Geometry check sheet. Reference: the model listing, model coordinates, mm. Give positions to 0.01 mm unless a question says otherwise; leave off trailing zeros. Loops run counter-clockwise (first coordinate to the right, second up) from the corner with the lowest first, then second, coordinate; pieces in that order, holes last. Notation, with made-up numbers: (86, 57) -> (136, 57) arc R31 ccw to (136, 89) -> close; hole circle Ø1 at (14, 29.5). An arc over 180 degrees is marked (long way). One line per question, with ' | ' between items.
from build123d import *

# Parameters (mm, degrees)
ESBO_O1_W                = 150
ESBO_O1_H                = 40
ESBO_O1_R                = 2.5
ESBO_O1_R_2              = 6
RESSALTO_EXTRUS_O1_DEPTH = 12.7
ESBO_O4_R                = 5.5
CORTE_EXTRUS_O1_DEPTH    = 8
ESBO_O7_W                = 150
ESBO_O7_H                = 10
RESSALTO_EXTRUS_O4_DEPTH = 12.7
ESBO_O8_W                = 10
ESBO_O8_H                = 50
RESSALTO_EXTRUS_O5_DEPTH = 12.7
ESBO_O9_R                = 2
CORTE_EXTRUS_O2_DEPTH    = 10


with BuildPart() as part:
    # Esboço1 → Ressalto-extrusão1 (new body)
    with BuildSketch(Plane(origin=(0, 0, 0), x_dir=(1, 0, 0), z_dir=(0, 1, 0))):
        Rectangle(ESBO_O1_W, ESBO_O1_H)
        with Locations(Location((0, 0, 0), (0, 0, 270))):
            Circle(ESBO_O1_R, mode=Mode.SUBTRACT)
        with Locations(Location((-57.5, 0, 0), (0, 0, 270))):
            Circle(ESBO_O1_R_2, mode=Mode.SUBTRACT)
        with Locations(Location((57.5, 0, 0), (0, 0, 270))):
            Circle(ESBO_O1_R_2, mode=Mode.SUBTRACT)
    extrude(amount=RESSALTO_EXTRUS_O1_DEPTH)

    # Esboço4 → Corte-extrusão1 (cut)
    with BuildSketch(Plane.XZ):
        with Locations(Location((0, 0, 0), (0, 0, 270))):
            Circle(ESBO_O4_R)
    extrude(amount=-CORTE_EXTRUS_O1_DEPTH, mode=Mode.SUBTRACT)

    # Esboço7 → Ressalto-extrusão4 (add)
    with BuildSketch(Plane.XZ):
        with Locations((0, 25)):
            Rectangle(ESBO_O7_W, ESBO_O7_H)
    extrude(amount=-RESSALTO_EXTRUS_O4_DEPTH)

    # Esboço8 → Ressalto-extrusão5 (add)
    with BuildSketch(Plane.XZ):
        with Locations((-80, 5)):
            Rectangle(ESBO_O8_W, ESBO_O8_H)
        with Locations((80, 5)):
            Rectangle(ESBO_O8_W, ESBO_O8_H)
    extrude(amount=-RESSALTO_EXTRUS_O5_DEPTH)

    # Esboço9 → Corte-extrusão2 (cut)
    with BuildSketch(Plane(origin=(85, 0, 0), x_dir=(0, 0, -1), z_dir=(1, 0, 0))):
        with Locations((0, 6.35)):
            Circle(ESBO_O9_R)
    corte_extrus_o2 = extrude(amount=-CORTE_EXTRUS_O2_DEPTH, mode=Mode.SUBTRACT)

    # Esboço13 → Furo roscado de M52 (revolve, cut)
    with BuildSketch(Plane(origin=(85, 6.35, 0), x_dir=(0, 0, -1), z_dir=(0, 1, 0))):
        Polygon((0, 0), (0, 30.2618073), (2.1, 29), (2.1, 5), (2.5, 5), (2.5, 0), align=None)
    furo_roscado_de_m52 = revolve(axis=Axis((91.35, 6.35, 0), (-1, 0, 0)), mode=Mode.SUBTRACT)

    # Espelhar1: Corte-extrusão2, Furo roscado de M52 across plane
    add(corte_extrus_o2.mirror(Plane(origin=(0, 0, 0), x_dir=(0, 0, 1), z_dir=(1, 0, 0))), mode=Mode.SUBTRACT)
    add(furo_roscado_de_m52.mirror(Plane(origin=(0, 0, 0), x_dir=(0, 0, 1), z_dir=(1, 0, 0))), mode=Mode.SUBTRACT)


solid = part.part
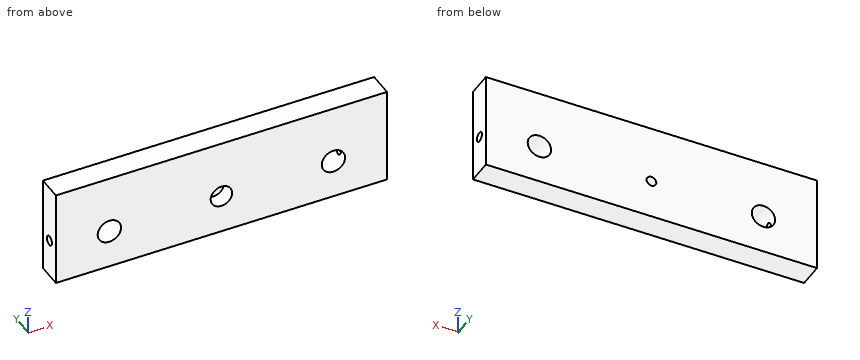
Item 1: Sectioned sample at A-A (x = -57.5). Record the cut outline in (y, z), plus the area to 3 significant figures.
Result:
outline: (0, -20) -> (12.7, -20) -> (12.7, -6) -> (0, -6) -> close; (0, 6) -> (12.7, 6) -> (12.7, 30) -> (0, 30) -> close | area: 483 mm2
Item 2: Sectioned sample at D-D (x = 0). Record the cut outline in (y, z), plus the area to 4 significant figures.
Result:
outline: (0, -20) -> (12.7, -20) -> (12.7, -2.5) -> (8, -2.5) -> (8, -5.5) -> (0, -5.5) -> close; (0, 5.5) -> (8, 5.5) -> (8, 2.5) -> (12.7, 2.5) -> (12.7, 30) -> (0, 30) -> close | area: 523.5 mm2
Item 3: Scan lines: probe 1 along X at (y, z) = (9.3, 0); probe 2 along X at (y, z) = (5.25, 0); probe 3 along Y at (x, z) = (82, 0). Record each from-to range of solid material in increasing order.
Result:
probe 1: -85 to -63.5, -51.5 to -2.5, 2.5 to 51.5, 63.5 to 85 | probe 2: -51.5 to -5.5, 5.5 to 51.5 | probe 3: 0 to 3.85, 8.85 to 12.7
Item 4: Sectioned sample at C-C (z = 0). Give the number of separate pieces and of enclosed holes in the cut face, plus the area to 3 significant figures.
Result:
separate pieces: 6 | enclosed holes: 0 | area: 1,550 mm2
Item 5: Sectioned sample at B-B (y = 6.35). Record the cut outline in (x, z).
Result:
outline: (-85, -20) -> (85, -20) -> (85, -2.5) -> (80, -2.5) -> (80, -2.1) -> (63.12, -2.1) arc R6 cw (long way) to (63.12, 2.1) -> (80, 2.1) -> (80, 2.5) -> (85, 2.5) -> (85, 30) -> (-85, 30) -> (-85, 2.5) -> (-80, 2.5) -> (-80, 2.1) -> (-63.12, 2.1) arc R6 cw (long way) to (-63.12, -2.1) -> (-80, -2.1) -> (-80, -2.5) -> (-85, -2.5) -> close; hole circle Ø11 at (0, 0)
Item 6: Depth check by flat-ended pin: pin 1 Ø4 at (y, z) = (6.35, 0) entering from +X; pin 2 Ø3.5 at (y, z) = (6.35, 0) entering from -X; pin 3 Ø5.5 at (x, z) = (0.5, -0.5) entering from -Y. Enter the tip coordinate at first touch or a pass-through.
Result:
pin 1: x = 51.84 | pin 2: x = -51.76 | pin 3: y = 8
